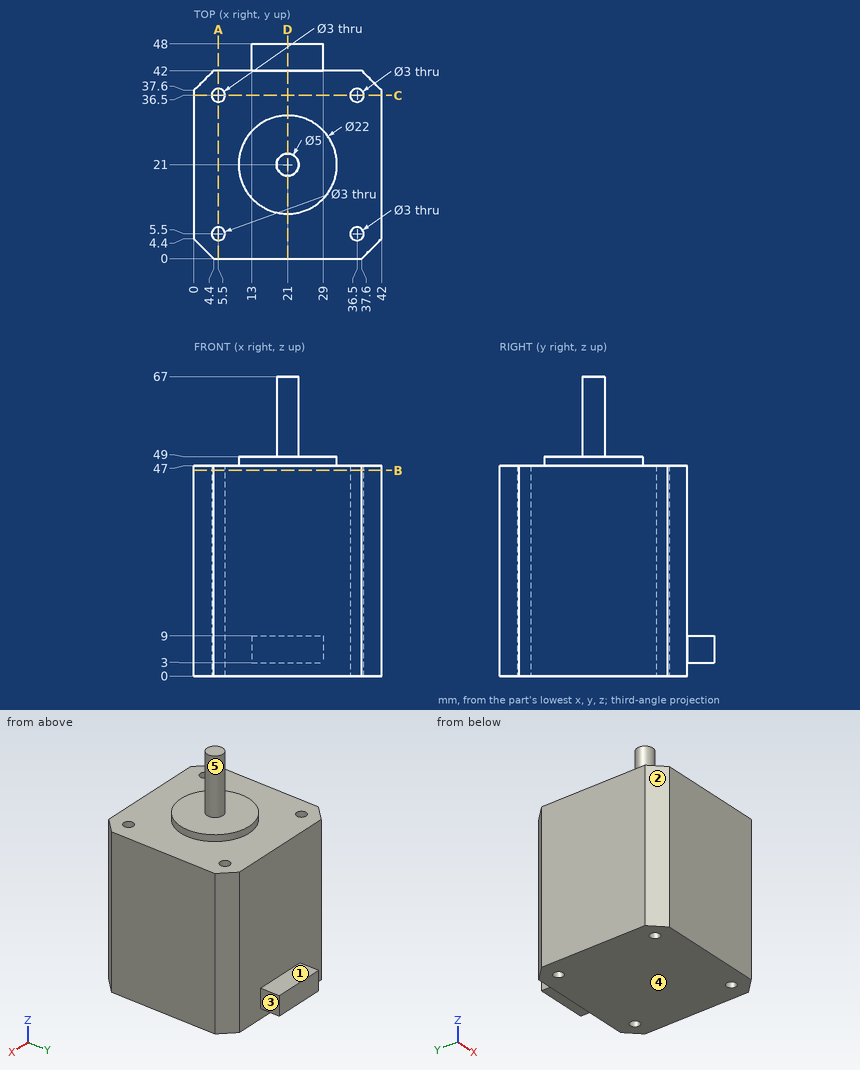
Verification items for this drawing (mm, ordinates from the low corner). A direction names the side the tool comes from. Give positions to 0.01 mm unless a question says otherwise; leave off trailing zeros. Loops run counter-clockwise (first coordinate to the right, second up) from the corner with the lowest first, then second, coordinate; pieces in that order, holes last.
1. Tool access check on the marked faces 1, 2, 3, 4 and 5. Record the directions out of +Z, -Z, +X, -X, +Y, -Y that give a thin tool (end or side, any length) a straight path to the whole face; none if there is none.
Derived:
face 1: +Z, +X, -X, +Y
face 2: +Z, -Z, -X, -Y
face 3: +Z, -Z, +X, +Y
face 4: -Z, +X, -X, +Y, -Y
face 5: +Z
2. Go/stop test with flat-tipped pins: P1, Ø10, axis at x = 27.5, z = 23, coming from the +Y side; P2, Ø10, axis at x = 17, y = 12, coming from the -Z side; P3, Ø1, axis at x = 8.5, y = 12, coming from the +Z side; P4, Ø6.5, axis at x = 16, y = 16, coming from the +Z side. Record where each tip stops, or that it passes through.
Derived:
P1: stops at y = 42
P2: stops at z = 0
P3: stops at z = 47
P4: stops at z = 49
3. Material ranges on probe 1 along Y at (x, z) = (5.5, 33.5); probe 2 along Y at (x, z) = (36, 27); probe 3 along Z at (x, y) = (9, 21), recorded low to high.
Derived:
probe 1: y = 0 to 4, 7 to 35, 38 to 42
probe 2: y = 0 to 4.09, 6.91 to 35.09, 37.91 to 42
probe 3: z = 0 to 47
4. Cross-section at B-B on z = 46. Record the cut outline in (x, y), and give its area (3 significant figures).
Derived:
outline: (0, 4.4) - (4.4, 0) - (37.6, 0) - (42, 4.4) - (42, 37.6) - (37.6, 42) - (4.4, 42) - (0, 37.6) - close; hole circle Ø3 at (5.5, 5.5); hole circle Ø3 at (5.5, 36.5); hole circle Ø3 at (36.5, 5.5); hole circle Ø3 at (36.5, 36.5)
area: 1,700 mm2
5. Cross-section at A-A on x = 5.5. Record the cut outline in (y, z).
Derived:
outline: (0, 0) - (4, 0) - (4, 47) - (0, 47) - close; (7, 0) - (35, 0) - (35, 47) - (7, 47) - close; (38, 0) - (42, 0) - (42, 47) - (38, 47) - close
6. Cross-section at D-D on x = 21. Record the cut outline in (y, z).
Derived:
outline: (0, 0) - (42, 0) - (42, 3) - (48, 3) - (48, 9) - (42, 9) - (42, 47) - (32, 47) - (32, 49) - (23.5, 49) - (23.5, 67) - (18.5, 67) - (18.5, 49) - (10, 49) - (10, 47) - (0, 47) - close
